Design review of the part built by this model. Coordinates are the model's own, in mm. Coordinates: 2 decimals unless noted, no trailing zeros. Write each loop counter-clockwise with the first axis right and the second up, starting at its lowest first coordinate (ties: lowest second). Pieces come first, ordered by that corner, then holes.
Q1. Take a section at B-B (z = -27). Give the boundary of the cut face in (x, y).
Q2. For probe 1 along Z at (x, y) = (6, 5); probe 2 along Y at (x, z) = (6, -135); probe 3 along Z at (x, y) = (1.75, 72), list the stretches that pass through material, from the lowest coordinate up.
Q3. Insertion check: pin 1 (1.9 mm diameter, centred on x = 3.5, y = 174.5, fed in from +Z); pin 2 (1.9 mm diameter, centred on x = 2, z = -98, fed in from -Y); pin 3 (2 mm diameter, centred on x = 5.5, y = 76.5, fed in from -Z); pin 4 (14.5 mm diameter, centred on y = 43.63, z = -42.71, fed in from +X). Each pin has a flat end and moves straight along its axis. Give the tip position at first contact, or say it passes through.
Q4. Take a section at A-A (x = 3.75). State how many separate pieces and enclosed holes the cut face has, and give its area (3 significant figures).
```python
from build123d import *

# Parameters (mm, degrees)
SKETCH1_R      = 12.049005967
SKETCH1_R_2    = 2.032
EXTRUDE1_DEPTH = 6.35
FILLET3_R      = 17.78
FILLET8_R      = 6.1976
FILLET10_R     = 6.35


with BuildPart() as part:
    # Sketch1 → Extrude1 (new body)
    with BuildSketch(Plane(origin=(0, 0, 0), x_dir=(0, 0, -1), z_dir=(1, 0, 0))):
        with BuildLine():
            Line((13.365344838, 110), (0, 110))
            add(Edge.make_bspline(
                [(23.525344838, 0), (23.886396453, 21.77280911), (16.984017385, 81.503501161), (0, 110)],
                knots=[0, 0, 0, 0, 1, 1, 1, 1], degree=3))
            Line((23.525344838, 0), (33.046497245, 0))
            Line((33.046497245, 0), (33.046497245, 10.25525))
            Line((33.046497245, 10.25525), (31.062122245, 10.25525))
            Line((31.062122245, 10.25525), (31.034086884, 14.224))
            Line((31.034086884, 14.224), (38.971586884, 14.224))
            Line((38.971586884, 14.224), (38.999622245, 10.25525))
            Line((38.999622245, 10.25525), (37.015247245, 10.25525))
            Line((37.015247245, 10.25525), (37.015247245, 0))
            Line((37.015247245, 0), (47.956836884, 0))
            Line((47.956836884, 0), (47.956836884, -6.858))
            Line((47.956836884, -6.858), (58.116836884, -6.858))
            Line((58.116836884, -6.858), (58.116836884, 0))
            Line((58.116836884, 0), (68.606497245, 0))
            Line((68.606497245, 0), (68.606497245, 10.25525))
            Line((68.606497245, 10.25525), (66.622122245, 10.25525))
            Line((66.622122245, 10.25525), (66.594086884, 14.224))
            Line((66.594086884, 14.224), (74.531586884, 14.224))
            Line((74.531586884, 14.224), (74.559622245, 10.25525))
            Line((74.559622245, 10.25525), (72.575247245, 10.25525))
            Line((72.575247245, 10.25525), (72.575247245, 0))
            Line((72.575247245, 0), (83.516836884, 0))
            Line((83.516836884, 0), (83.516836884, -6.858))
            Line((83.516836884, -6.858), (93.676836884, -6.858))
            Line((93.676836884, -6.858), (93.676836884, 0))
            Line((93.676836884, 0), (106.68, 0))
            ThreePointArc((106.68, 0), (147.01715629, 48.348482811), (159.813733796, 110))
            Line((159.813733796, 110), (152.578339639, 110))
            Line((152.578339639, 110), (152.578339639, 99.96875))
            Line((152.578339639, 99.96875), (154.562714639, 99.96875))
            Line((154.562714639, 99.96875), (154.59075, 96))
            Line((154.59075, 96), (146.65325, 96))
            Line((146.65325, 96), (146.625214639, 99.96875))
            Line((146.625214639, 99.96875), (148.609589639, 99.96875))
            Line((148.609589639, 99.96875), (148.609589639, 110))
            Line((148.609589639, 110), (137.922, 110))
            Line((137.922, 110), (137.922, 116.858))
            Line((137.922, 116.858), (127.762, 116.858))
            Line((127.762, 116.858), (127.762, 110))
            Line((127.762, 110), (117.018339639, 110))
            Line((117.018339639, 110), (117.018339639, 99.74475))
            Line((117.018339639, 99.74475), (119.002714639, 99.74475))
            Line((119.002714639, 99.74475), (119.03075, 95.776))
            Line((119.03075, 95.776), (111.09325, 95.776))
            Line((111.09325, 95.776), (111.065214639, 99.74475))
            Line((111.065214639, 99.74475), (113.049589639, 99.74475))
            Line((113.049589639, 99.74475), (113.049589639, 110))
            Line((113.049589639, 110), (97.632376997, 110))
            add(Edge.make_bspline(
                [(97.632376997, 110), (102.845891428, 148.686045998), (104.019096982, 168.115161248), (100.196457803, 179.300454229)],
                knots=[0.263690297, 0.263690297, 0.263690297, 0.263690297, 1, 1, 1, 1], degree=3))
            Line((100.196457803, 179.300454229), (100.196457803, 186.158454229))
            Line((100.196457803, 186.158454229), (90.036457803, 186.158454229))
            Line((90.036457803, 186.158454229), (90.036457803, 179.300454229))
            Line((90.036457803, 179.300454229), (79.292797442, 179.300454229))
            Line((79.292797442, 179.300454229), (79.292797442, 169.045204229))
            Line((79.292797442, 169.045204229), (81.277172442, 169.045204229))
            Line((81.277172442, 169.045204229), (81.305207803, 165.076454229))
            Line((81.305207803, 165.076454229), (73.367707803, 165.076454229))
            Line((73.367707803, 165.076454229), (73.339672442, 169.045204229))
            Line((73.339672442, 169.045204229), (75.324047442, 169.045204229))
            Line((75.324047442, 169.045204229), (75.324047442, 179.300454229))
            Line((75.324047442, 179.300454229), (64.636457803, 179.300454229))
            Line((64.636457803, 179.300454229), (64.636457803, 186.158454229))
            Line((64.636457803, 186.158454229), (54.476457803, 186.158454229))
            add(Edge.make_bspline(
                [(54.476457803, 186.158454229), (63.233505027, 173.481312137), (60.112941012, 141.740656068), (56.992376997, 110)],
                knots=[0, 0, 0, 0, 1, 1, 1, 1], degree=3))
            Line((56.992376997, 110), (38.181684477, 110))
            Line((38.181684477, 110), (38.181684477, 99.74475))
            Line((38.181684477, 99.74475), (40.166059477, 99.74475))
            Line((40.166059477, 99.74475), (40.194094838, 95.776))
            Line((40.194094838, 95.776), (32.256594838, 95.776))
            Line((32.256594838, 95.776), (32.228559477, 99.74475))
            Line((32.228559477, 99.74475), (34.212934477, 99.74475))
            Line((34.212934477, 99.74475), (34.212934477, 110))
            Line((34.212934477, 110), (23.525344838, 110))
            Line((23.525344838, 110), (23.525344838, 116.858))
            Line((23.525344838, 116.858), (13.365344838, 116.858))
            Line((13.365344838, 116.858), (13.365344838, 110))
        make_face()
        Polygon((77.081007641, 31.622417606), (82.911687358, 35.23286606), (88.260499882, 26.594822035), (82.429820165, 22.984373581), align=None, mode=Mode.SUBTRACT)
        with Locations((42.714261702, 43.633986225)):
            Circle(SKETCH1_R, mode=Mode.SUBTRACT)
        with Locations((73.310331844, 44.225196864)):
            Circle(SKETCH1_R_2, mode=Mode.SUBTRACT)
        Polygon((139.194257476, 46.072756303), (132.336275936, 46.056844127), (132.312702342, 56.216816779), (139.170683882, 56.232728955), align=None, mode=Mode.SUBTRACT)
        Polygon((58.360163805, 61.855571693), (64.190843522, 65.466020147), (69.539656047, 56.827976122), (63.70897633, 53.217527668), align=None, mode=Mode.SUBTRACT)
        with BuildLine():
            ThreePointArc((106.081947056, 79.295723893), (108.313793383, 84.683877565), (113.701947056, 86.915723893))
            Line((113.701947056, 86.915723893), (117.511947056, 86.915723893))
            ThreePointArc((117.511947056, 86.915723893), (122.900100729, 84.683877565), (125.131947056, 79.295723893))
            Line((125.131947056, 79.295723893), (125.131947056, 56.435723893))
            ThreePointArc((125.131947056, 56.435723893), (122.900100729, 51.04757022), (117.511947056, 48.815723893))
            Line((117.511947056, 48.815723893), (113.701947056, 48.815723893))
            ThreePointArc((113.701947056, 48.815723893), (108.313793383, 51.04757022), (106.081947056, 56.435723893))
            Line((106.081947056, 56.435723893), (106.081947056, 79.295723893))
        make_face(mode=Mode.SUBTRACT)
        with Locations((54.589488008, 74.458350952)):
            Circle(SKETCH1_R_2, mode=Mode.SUBTRACT)
        with Locations((135.765266706, 68.924861749)):
            Circle(SKETCH1_R_2, mode=Mode.SUBTRACT)
        with BuildLine():
            ThreePointArc((56.974437356, 89.423104749), (56.03531954, 95.179092566), (59.441360982, 99.913247161))
            Line((59.441360982, 99.913247161), (62.214897914, 101.630664789))
            ThreePointArc((62.214897914, 101.630664789), (67.970885731, 102.569782605), (72.705040326, 99.163741163))
            Line((72.705040326, 99.163741163), (91.425884161, 68.930587076))
            ThreePointArc((91.425884161, 68.930587076), (92.365001978, 63.174599258), (88.958960536, 58.440444664))
            Line((88.958960536, 58.440444664), (86.185423604, 56.723027036))
            ThreePointArc((86.185423604, 56.723027036), (80.429435786, 55.783909219), (75.695281192, 59.189950661))
            Line((75.695281192, 59.189950661), (56.974437356, 89.423104749))
        make_face(mode=Mode.SUBTRACT)
        Polygon((139.170683882, 81.616994542), (132.312702342, 81.632906718), (132.336275936, 91.79287937), (139.194257476, 91.776967194), align=None, mode=Mode.SUBTRACT)
    extrude(amount=EXTRUDE1_DEPTH)

    # Fillet3
    fillet3_edges = [part.edges().sort_by_distance(p)[0] for p in [
        (3.175, 0, -106.68),
    ]]
    fillet(fillet3_edges, radius=FILLET3_R)

    # Fillet8
    fillet8_edges = [part.edges().sort_by_distance(p)[0] for p in [
        (3.175, 186.158454229, -54.476457803),
    ]]
    fillet(fillet8_edges, radius=FILLET8_R)

    # Fillet10
    fillet10_edges = [part.edges().sort_by_distance(p)[0] for p in [
        (3.175, 186.158454229, -100.196457803),
    ]]
    fillet(fillet10_edges, radius=FILLET10_R)


solid = part.part
```
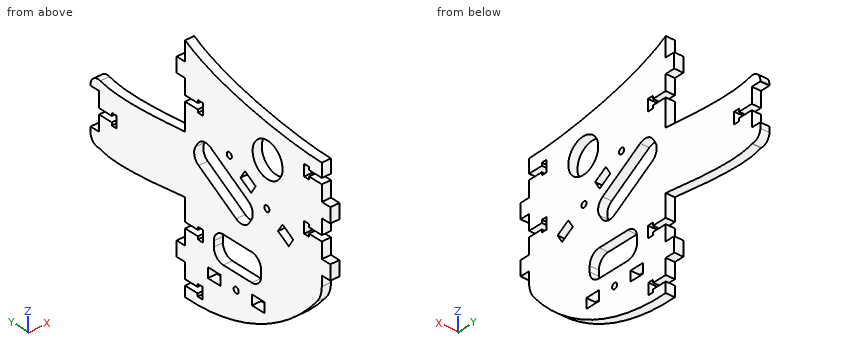
Response:
1. outline: (0, 0) - (6.35, 0) - (6.35, 110) - (0, 110) - close
2. probe 1: z = -113.1 to -72.58, -68.61 to -37.02, -33.05 to -23.5
2. probe 2: y = 28.31 to 46.06, 56.22 to 67.04, 70.81 to 81.63, 91.79 to 116.86
2. probe 3: z = -155.72 to -125.13, -106.08 to -89.53, -67.76 to -14.14
3. pin 1: stops at z = -58.61
3. pin 2: stops at y = 0
3. pin 3: stops at z = -157.03
3. pin 4: passes through
4. separate pieces: 1
4. enclosed holes: 10
4. area: 14,700 mm2
